```python
from build123d import *
from build123d.topology import SkipClean

# Parameters (mm, degrees)
SKETCH_1_R               = 5
SKETCH_1_W               = 40
SKETCH_1_H               = 6
EXTRUDE_1_DEPTH          = 2
CUT_EXTRUDE_2_DEPTH      = 46.44227107
CUT_EXTRUDE_2_DEPTH_BACK = 46.44227107
SKETCH_1_3_R             = 2
FILLET_1_R               = 3
EXTRUDE_START            = -1
EXTRUDE_2_DEPTH          = 1
SKETCH_2_R               = 2
EXTRUDE_3_DEPTH          = 6
SKETCH_2_3_R             = 1.8
EXTRUDE_4_DEPTH          = 4
EXTRUDE_START_2          = -10
SKETCH_2_4_R             = 1.8
EXTRUDE_5_DEPTH          = 4


with BuildPart() as part:
    # 草图1 → 凸台-拉伸1 (new body)
    with BuildSketch(Plane(origin=(0, 0, 0), x_dir=(0, 0, -1), z_dir=(1, 0, 0))):
        Circle(SKETCH_1_R)
        with Locations((40, -1)):
            Circle(SKETCH_1_R)
        with Locations((20, 0)):
            Rectangle(SKETCH_1_W, SKETCH_1_H)
    extrude(amount=EXTRUDE_1_DEPTH)

    # 草图1<3> → 切除-拉伸2 (cut, two sides: drawn at the far end of the back side and taken through both)
    with BuildSketch(Plane(origin=(0, 0, 0), x_dir=(0, 0, -1), z_dir=(1, 0, 0)).offset(-CUT_EXTRUDE_2_DEPTH_BACK)):
        Circle(SKETCH_1_3_R)
        with Locations((40, -1)):
            Circle(SKETCH_1_3_R)
    extrude(amount=CUT_EXTRUDE_2_DEPTH + CUT_EXTRUDE_2_DEPTH_BACK, mode=Mode.SUBTRACT)

    # 圆角1
    fillet_1_edges = [part.edges().sort_by_distance(p)[0] for p in [
        (1, -3, -35.417424305),
        (1, 3, -37),
        (1, 3, -4),
        (1, -3, -4),
    ]]
    fillet(fillet_1_edges, radius=FILLET_1_R)

    # 草图1<4> → 凸台-拉伸2 (add)
    with SkipClean():  # the faces are left unmerged after this step: merging them gives an invalid solid
        with BuildSketch(Plane(origin=(0, 0, 0), x_dir=(0, 0, -1), z_dir=(1, 0, 0)).offset(EXTRUDE_START)):
            with BuildLine():
                ThreePointArc((37, 3), (35.16534763, 0.275200556), (35.417424305, -3))
                Line((35.417424305, -3), (40, -3))
                ThreePointArc((40, -3), (38, -1), (40, 1))
                Line((40, 1), (40, 3))
                Line((40, 3), (37, 3))
            make_face()
            with BuildLine():
                Line((40, -3), (35.417424305, -3))
                ThreePointArc((35.417424305, -3), (41.021548218, -5.894531565), (45, -1))
                ThreePointArc((45, -1), (42.236067977, 3.472135955), (37, 3))
                Line((37, 3), (40, 3))
                Line((40, 3), (40, 1))
                ThreePointArc((40, 1), (41.414213562, 0.414213562), (42, -1))
                ThreePointArc((42, -1), (41.414213562, -2.414213562), (40, -3))
            make_face()
        extrude(amount=EXTRUDE_2_DEPTH)

    # 镜向3: part across plane


with BuildPart() as part_1:
    add(part.part)
    add(part.part.mirror(Plane.ZY.offset(1)))

    # 草图2 → 凸台-拉伸3 (add)
    with BuildSketch(Plane(origin=(2, 0, 0), x_dir=(0, 0, -1), z_dir=(1, 0, 0))):
        with Locations((40, -1)):
            Circle(SKETCH_2_R)
    extrude(amount=-EXTRUDE_3_DEPTH)

    # 草图2<3> → 凸台-拉伸4 (add)
    with BuildSketch(Plane(origin=(2, 0, 0), x_dir=(0, 0, -1), z_dir=(1, 0, 0))):
        with Locations((40, -1)):
            Circle(SKETCH_2_3_R)
    extrude(amount=EXTRUDE_4_DEPTH)

    # 草图2<4> → 凸台-拉伸5 (add)
    with BuildSketch(Plane(origin=(2, 0, 0), x_dir=(0, 0, -1), z_dir=(1, 0, 0)).offset(EXTRUDE_START_2)):
        with Locations((40, -1)):
            Circle(SKETCH_2_4_R)
    extrude(amount=EXTRUDE_5_DEPTH)


solid = part_1.part
```
Source: CAD feature listing. Evaluate the final solid. Frame: model axes, mm. A direction names the side the tool comes from. Round coordinates to 2 decimals unless told otherwise and drop trailing zeros. Loops run counter-clockwise (first coordinate to the right, second up) from the corner with the lowest first, then second, coordinate; pieces in that order, holes last. Notation, with made-up numbers: M 76.25,13 L 97.25,13 A26 cw 97.25,29 Z; hole C 54.5,-23 d1. An arc over 180 degrees is marked long. Use a Markdown table: item, result. Add a question column.
1. Reachability of faces 5 (the flat face through (-3, 3, -20)), 6 (the cylindrical face through (-3.014, -3.188, -4.245)), 7 (the flat face through (-8, -1, -40)) from +Z, -Z, +X, -X, +Y, -Y: full face, straight path, thin tool, end or side. Return the list, or none.
2. Contact query for flat-ended pins moving along their axis: P1, Ø1.6, axis at x = 1.5, z = -16.5, coming from the +Y side; P2, Ø3, axis at y = 1.5, z = -17, coming from the +X side; P3, Ø5, axis at x = -0.5, z = -7.5, coming from the -Y side. Output: stop coordinate, or through.
3. Mould query, pull axis Z, two halves, no side actions, for faces 1 (the flat face through (-3, -3, -19)), 2 (the cylindrical face through (1.01, -3.29, -35.04)), 3 (the flat face through (6, -1, -40)), 4 (the cylindrical face through (3.972, -0.459, -41.717)). Classes: pulls with the +Z half, pulls with the -Z half, needs draft (parallel to the pull), parting line crosses it, or undercut.
4. Section query C-C on z = -21. Return the cut outline in (x, y), then the cut area to 3 significant figures.
5. Section query B-B on z = 0. Return the cut outline in (x, y).
6. Section query D-D on y = -1.5. Return the cut outline in (x, z).
7. Line query: line 1 (X direction, y = -1.5, z = -2.5); line 2 (Y direction, x = -3.25, z = 0); line 3 (Z direction, x = -3.25, y = -3.75). Output: solid intervals per line, ascending.
Reported:
| question | item | result |
|---|---|---|
| 1 | face 5 | +X, -X, +Y |
| 1 | face 6 | +X, -X, -Y |
| 1 | face 7 | +Z, -Z, -X, +Y, -Y |
| 2 | P1 | stops at y = 3 |
| 2 | P2 | stops at x = 2 |
| 2 | P3 | stops at y = -3.01 |
| 3 | face 1 | undercut |
| 3 | face 2 | undercut |
| 3 | face 3 | needs draft |
| 3 | face 4 | parting line crosses it |
| 4 | outline | M -4,-3 L -2,-3 L -2,3 L -4,3 Z; M 0,-3 L 2,-3 L 2,3 L 0,3 Z |
| 4 | area | 24.0 mm² |
| 5 | outline | M -4,-5 L -2,-5 L -2,-2 L -4,-2 Z; M -4,2 L -2,2 L -2,5 L -4,5 Z; M 0,-5 L 2,-5 L 2,-2 L 0,-2 Z; M 0,2 L 2,2 L 2,5 L 0,5 Z |
| 6 | outline | M -8,-41.73 L -4,-41.73 L -4,-44.97 L 2,-44.97 L 2,-41.73 L 6,-41.73 L 6,-38.27 L 2,-38.27 L 2,-1.32 L 0,-1.32 L 0,-35.03 L -2,-35.03 L -2,-1.32 L -4,-1.32 L -4,-38.27 L -8,-38.27 Z; M -4,1.32 L -2,1.32 L -2,4.77 L -4,4.77 Z; M 0,1.32 L 2,1.32 L 2,4.77 L 0,4.77 Z |
| 7 | line 1 | x = -4 to -2, 0 to 2 |
| 7 | line 2 | y = -5 to -2, 2 to 5 |
| 7 | line 3 | z = -44.18 to -35.74, -3.31 to 3.31 |
